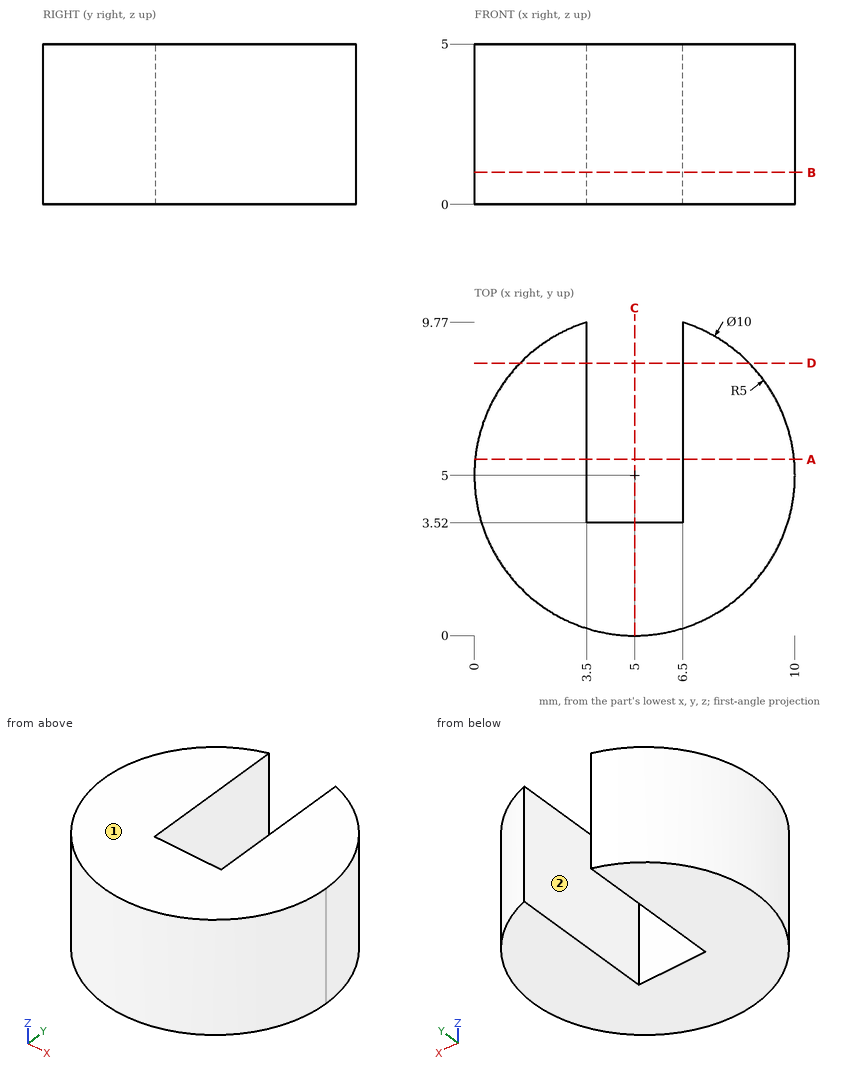
Study the drawing (mm; zero at the part's minimum x, y, z) and answer. A direction names the side the tool comes from. Give positions to 0.01 mm unless a question says otherwise; leave off trailing zeros. Loops run counter-clockwise (first coordinate to the right, second up) from the corner with the lowest first, then second, coordinate; pieces in that order, holes last. Notation, with made-up numbers: M 0,-37.5 L 7,-37.5 A27 cw 7,-15.5 Z; hole C 55,72.5 d7. An arc over 180 degrees is marked long. Answer as CSV lines item,"result".
Item 1: Which of the six approach directions +Z, -Z, +X, -X, +Y, -Y give full straight-line access (tool end or side, diameter ignored) to the marked faces 1 and 2?
Values follow:
face 1,"+Z, +X, -X, +Y, -Y"
face 2,"+Z, -Z, +Y"
Item 2: The part is cut by section C-C (x = 5). Give the vertices of the cut face in (y, z).
Values follow:
outline,"M 0,0 L 3.52,0 L 3.52,5 L 0,5 Z"
Item 3: The part is cut by section D-D (y = 8.5). Give the vertices of the cut face in (x, z).
Values follow:
outline,"M 1.43,0 L 3.5,0 L 3.5,5 L 1.43,5 Z; M 6.5,0 L 8.57,0 L 8.57,5 L 6.5,5 Z"
Item 4: The part is cut by section A-A (y = 5.5). Give the vertices of the cut face in (x, z) (1 decimal).
Values follow:
outline,"M 0,0 L 3.5,0 L 3.5,5 L 0,5 Z; M 6.5,0 L 10,0 L 10,5 L 6.5,5 Z"
Item 5: Given pin 1 Ø2 at (x, z) = (9, 2) entering from +Y, flat-ended and moving along its own axis, determine where the tip first touches the part or whether it passes through.
Values follow:
pin 1,"stops at y = 9"
Item 6: The part is cut by section B-B (z = 1). Give the vertices of the cut face in (x, y).
Values follow:
outline,"M 3.5,3.52 L 3.5,9.77 A5 ccw long 6.5,9.77 L 6.5,3.52 Z"
Item 7: Straight lines are drawn through the part: line 1 along Y through (x, z) = (5, 0.65); line 2 along X through (y, z) = (8, 4.8); line 3 along X through (y, z) = (8.25, 1.5). For each, find the intervals that lie inside material, in ascending order. Write a range as [from, to].
Values follow:
line 1,"y = [0, 3.52]"
line 2,"x = [1, 3.5], [6.5, 9]"
line 3,"x = [1.2, 3.5], [6.5, 8.8]"
